Can you work these out from the drawing? Everything is in mm from the part's minimum corner. A direction names the side the tool comes from. Coordinates: 2 decimals unless noted, no trailing zeros. Loops run counter-clockwise (first coordinate to the right, second up) from the corner with the lowest first, then second, coordinate; pieces in that order, holes last. Notation, with made-up numbers: (74.5, 54) - (132.5, 54) arc R16 cw to (132.5, 65) - close; hole circle Ø8 at (37.25, 51.25). An arc over 180 degrees is marked (long way). One line per question, with ' | ' between items. Start each with the question number.
1. I want a section at D-D, the plane x = 2.75. Write out the boundary of the cut face in (y, z), then the cut area to 3 significant figures.
2. I want a section at B-B, the plane y = 4.5. Write out the boundary of the cut face in (x, z).
3. Which directions (+Z, -Z, +X, -X, +Y, -Y) give clear straight access to the entire face, cutting with the end or side of a thin tool? Please do the marked faces 1, 2, 3, 4 and 5.
4. Please list where these lines run through material, in increasing order: L1, parallel to Z at x = 5.75, y = 2.5; L2, parallel to Z at x = 1.75, y = 3; L3, parallel to Y at x = 6.25, z = 19.5. Write a range as [from, to].
5. I'm going to push flat-ended pins straight in: P1, Ø1.2, axis at x = 0.5, z = 11.5, coming from the -Y side; P2, Ø1.9, axis at x = 4, z = 13.5, coming from the -Y side; P3, Ø1.4, axis at y = 2.5, z = 20, coming from the +X side. Where does each tip first touch, or does it pass through?
6. I want a section at A-A, the plane x = 4.2. Write out the boundary of the cut face in (y, z), then the cut area to 3 significant figures.
7. We'd pull the mould along Z, two halves only. Please class the marked faces 6, 7 and 8: pulls with the +Z half, pulls with the -Z half, needs draft (parallel to the pull), parting line crosses it, or undercut.
8. I want a section at C-C, the plane z = 7.15. Write out the boundary of the cut face in (x, y), then the cut area to 4 significant figures.
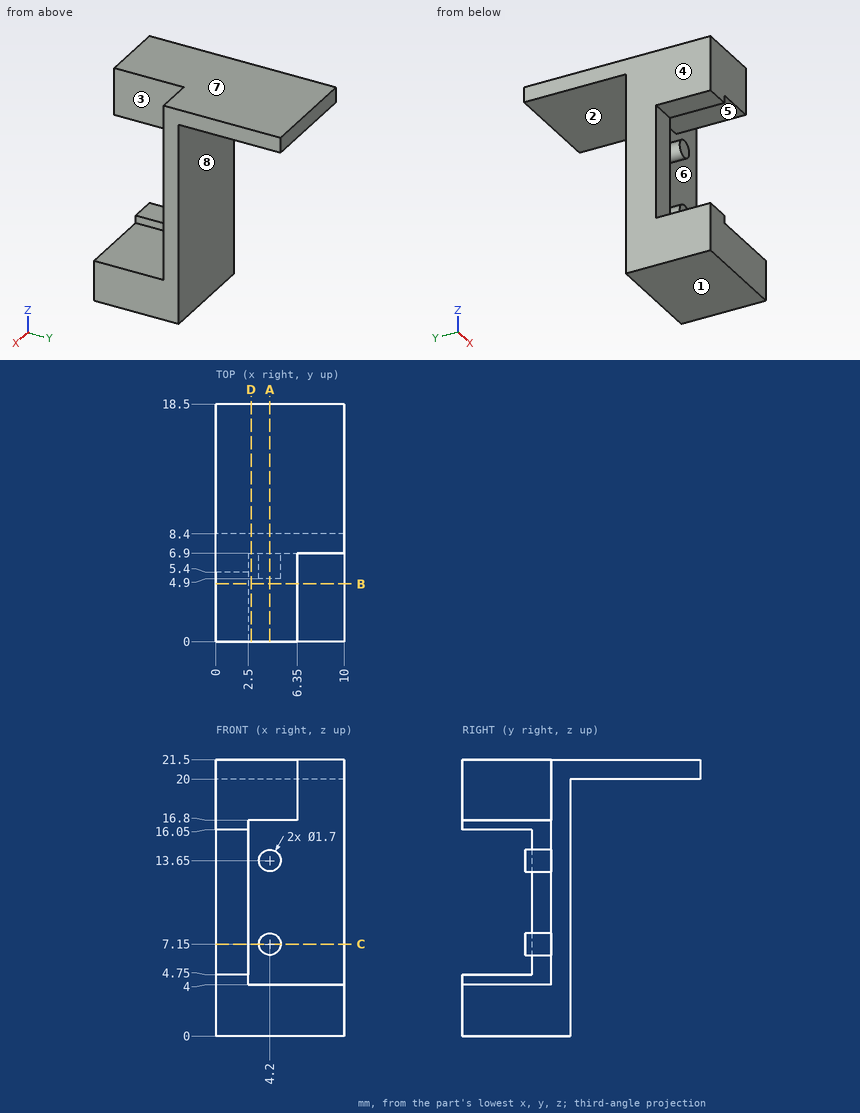
Results are:
1) outline: (0, 0) - (8.4, 0) - (8.4, 20) - (18.5, 20) - (18.5, 21.5) - (0, 21.5) - (0, 16.8) - (6.9, 16.8) - (6.9, 4) - (0, 4) - close | area: 107 mm2
2) outline: (0, 0) - (10, 0) - (10, 4) - (2.5, 4) - (2.5, 4.75) - (0, 4.75) - close; (0, 16.05) - (2.5, 16.05) - (2.5, 16.8) - (6.35, 16.8) - (6.35, 21.5) - (0, 21.5) - close
3) face 1: -Z, +X, -X, +Y, -Y | face 2: -Z, +X, -X, +Y | face 3: +Z, +X, -Y | face 4: +Z, -Z, -X, +Y, -Y | face 5: +X, -Y
4) L1: z = [0, 4], [16.8, 21.5] | L2: z = [0, 4.75], [16.05, 21.5] | L3: y = [0, 8.4]
5) P1: stops at y = 5.4 | P2: stops at y = 4.9 | P3: stops at x = 6.35
6) outline: (0, 0) - (8.4, 0) - (8.4, 20) - (18.5, 20) - (18.5, 21.5) - (0, 21.5) - (0, 16.8) - (6.9, 16.8) - (6.9, 14.5) - (4.9, 14.5) - (4.9, 12.8) - (6.9, 12.8) - (6.9, 8) - (4.9, 8) - (4.9, 6.3) - (6.9, 6.3) - (6.9, 4) - (0, 4) - close | area: 114 mm2
7) face 6: undercut | face 7: pulls with the +Z half | face 8: needs draft
8) outline: (0, 5.4) - (2.5, 5.4) - (2.5, 6.9) - (3.35, 6.9) - (3.35, 4.9) - (5.05, 4.9) - (5.05, 6.9) - (10, 6.9) - (10, 8.4) - (0, 8.4) - close | area: 22.15 mm2
